from build123d import *

# Parameters (mm, degrees)
PAD_DEPTH       = 7
SKETCH001_W     = 9
SKETCH001_H     = 4.46
POCKET_DEPTH    = 5
FILLET_R        = 0.3
SKETCH002_R     = 1.45
POCKET001_DEPTH = 3


with BuildPart() as part:
    # Sketch → Pad (new body)
    with BuildSketch(Plane.XY):
        with BuildLine():
            Line((-3.5, -2.5), (3.5, -2.5))
            Line((3.5, -2.5), (3.5, 2.5))
            Line((3.5, 2.5), (-3.5, 2.5))
            ThreePointArc((-3.5, 2.5), (-6.23383, 0), (-3.5, -2.5))
        make_face()
    extrude(amount=PAD_DEPTH)

    # Sketch001 (on DatumPlane) → Pocket (cut)
    with BuildSketch(Plane.XY.offset(7)):
        with Locations((2, -0.74)):
            Rectangle(SKETCH001_W, SKETCH001_H)
    extrude(amount=-POCKET_DEPTH, mode=Mode.SUBTRACT)

    # Fillet
    fillet_edges = [part.edges().sort_by_distance(p)[0] for p in [
        (0, -2.5, 0),
    ]]
    fillet(fillet_edges, radius=FILLET_R)

    # Sketch002 (on DatumPlane) → Pocket001 (cut)
    with BuildSketch(Plane.XY.offset(2)):
        with Locations((-0.5, -0.35)):
            Circle(SKETCH002_R)
    extrude(amount=-POCKET001_DEPTH, mode=Mode.SUBTRACT)


solid = part.part
Geometry: final body of the model. Coordinates: model frame, mm. A direction names the side the tool comes from. Give positions to 0.01 mm unless a question says otherwise; leave off trailing zeros. Loops run counter-clockwise (first coordinate to the right, second up) from the corner with the lowest first, then second, coordinate; pieces in that order, holes last. Notation, with made-up numbers: (26, -40) -> (50, -40) arc R32 cw to (50, -10) -> close; hole circle Ø4 at (61.5, -3). An arc over 180 degrees is marked (long way). Put each result on its own line as item: value.
1. Cut plane C-C (y = 0). Return the cut outline in (x, z), plus the area to 3 significant figures.
Taken from the geometry:
outline: (-6.23, 0.3) arc R0.3 ccw to (-5.93, 0) -> (-1.91, 0) -> (-1.91, 2) -> (-2.5, 2) -> (-2.5, 7) -> (-6.23, 7) -> close; (0.91, 0) -> (3.5, 0) -> (3.5, 2) -> (0.91, 2) -> close
area: 32.5 mm2
2. Ray query, line 1 along Y through (x, z) = (-0.5, 1.35); line 2 along Y through (x, z) = (3.25, 3.75); line 3 along Y through (x, z) = (-2.75, 1.25). Return the intervals inside material, ascending. Write a range as [from, to].
Taken from the geometry:
line 1: y = [-2.5, -1.8], [1.1, 2.5]
line 2: y = [1.49, 2.5]
line 3: y = [-2.5, 2.5]
3. Pull-direction query (Y, two-part tool) for faces 1 (the flat face through (-2.3, 0, 0)), 2 (the cylindrical face through (-1.65, -1.23, 1.01)), 3 (the flat face through (-1.1, -2.5, 1.6)); classes: released by +Y, released by -Y, zero draft, split by the parting line, or undercut.
Taken from the geometry:
face 1: zero draft
face 2: undercut
face 3: released by -Y
4. Pin query (flat end, axial travel): P1, Ø1.5, axis at x = -1.5, z = 4.5, coming from the +Y side; P2, Ø3, axis at y = -1, z = 5.5, coming from the +X side; P3, Ø2.5, axis at x = -0.5, z = 4, coming from the -Y side. Return the tip coordinate at first contact, or that it passes through.
Taken from the geometry:
P1: stops at y = 2.5
P2: stops at x = -2.5
P3: stops at y = 1.49
5. Cut plane A-A (x = 0.5). Return the cut outline in (y, z), plus the area to 3 significant figures.
Taken from the geometry:
outline: (-2.5, 0.3) arc R0.3 ccw to (-2.2, 0) -> (-1.4, 0) -> (-1.4, 2) -> (-2.5, 2) -> close; (0.7, 0) -> (2.2, 0) arc R0.3 ccw to (2.5, 0.3) -> (2.5, 7) -> (1.49, 7) -> (1.49, 2) -> (0.7, 2) -> close
area: 10.8 mm2
6. Cut plane B-B (z = 1.75). Return the cut outline in (x, y), plus the area to 3 significant figures.
Taken from the geometry:
outline: (-3.5, -2.5) -> (3.5, -2.5) -> (3.5, 2.5) -> (-3.5, 2.5) arc R2.51 ccw (long way) to start; hole circle Ø2.9 at (-0.5, -0.35)
area: 39.4 mm2
7. Set-up query: faces 4 (the flat face through (0, 2.5, 4)), 5 (the flat face through (-3, 1, 7)), 6 (the flat face through (1.1, -0.5, 2)). Return all of +Z, -Z, +X, -X, +Y, -Y with unobstructed straight access to the full face (end or side cutting, diameter ignored); none if empty.
Taken from the geometry:
face 4: +Z, -Z, +X, +Y
face 5: +Z, +X, -X, +Y, -Y
face 6: +Z, +X, -Y
8. Cut plane D-D (x = -2.25). Return the cut outline in (y, z), plus the area to 3 significant figures.
Taken from the geometry:
outline: (-2.5, 0.3) arc R0.3 ccw to (-2.2, 0) -> (2.2, 0) arc R0.3 ccw to (2.5, 0.3) -> (2.5, 7) -> (1.49, 7) -> (1.49, 2) -> (-2.5, 2) -> close
area: 15.0 mm2
